Model file for the job. Use its own axes, mm. A direction names the side the tool comes from. Give positions to 0.01 mm unless a question says otherwise; leave off trailing zeros. Loops run counter-clockwise (first coordinate to the right, second up) from the corner with the lowest first, then second, coordinate; pieces in that order, holes last. Notation, with made-up numbers: M 27.25,22 L 59.25,22 A17 ccw 59.25,34 Z; hole C 5,59.25 d2. An arc over 180 degrees is marked long. Use CSV: the item, a comma, the result in double quotes. Start each with the question number.
(1) Slice it at A-A on x = -44.5. List the corners of the cut face in (y, z).
(2) Tool access for faces 1 (the face through (-17, 8, 38.069)), 2 (the face through (0, 10, -17)), 3 (the face through (-17, 11, -9.431)): list every direction of +Z, -Z, +X, -X, +Y, -Y with a clear straight run to the whole face (end or side of a thin tool).
(3) Slice it at B-B on y = 3. List the corners of the cut face in (x, z).
(4) Slice it at C-C on z = 2. List the corners of the cut face in (x, y), and give its area (3 significant figures).
(5) Flat gauge pins, fed straight in: P1, Ø6, axis at x = -45, y = 6, coming from the -Z side; P2, Ø1.2, axis at x = -16.5, z = -10.5, coming from the +Y side; P3, Ø8, axis at x = -31.5, z = -4, coming from the -Y side. Where does each tip first touch, or does it go through?
(6) Wall check: line 1 along X through (y, z) = (6.75, 35.5); line 2 along Z through (x, y) = (-50, 10.5); line 3 along Y through (x, z) = (1, 20). Give the ranges that are in metal, low to high. Write a range as from..to.
(7) Two-plate mould, pull along Z, no slides. Class faces 4 (the face through (-17, 0, 8)), 5 (the face through (-17, 8, -21.931)), 6 (the face through (-17, 11, 13.069)): pulls with the +Z half, pulls with the -Z half, needs draft (parallel to the pull), parting line crosses it, or undercut.
(8) Slice it at D-D on x = -16. List the corners of the cut face in (y, z), and give its area (3 significant figures).
```python
from build123d import *

# Parameters (mm, degrees)
CROQUIS1_W                = 10
CROQUIS1_H                = 60
SALIENTE_EXTRUIR1_DEPTH   = 10
SALIENTE_EXTRUIR1_2_DEPTH = 10
SALIENTE_EXTRUIR1_3_DEPTH = 10
CROQUIS2_W                = 80
CROQUIS2_H                = 10
SALIENTE_EXTRUIR2_DEPTH   = 2.5


with BuildPart() as part:
    # Croquis1 → Saliente-Extruir1 (new body)
    with BuildSketch(Plane(origin=(0, 0, 0), x_dir=(1, 0, 0), z_dir=(0, 1, 0))):
        with Locations((-51.849391859, -8.068789191)):
            Rectangle(CROQUIS1_W, CROQUIS1_H)
    extrude(amount=SALIENTE_EXTRUIR1_DEPTH)



with BuildPart() as body_2:
    # Croquis1 → Saliente-Extruir1 2 (new body)
    with BuildSketch(Plane(origin=(0, 0, 0), x_dir=(1, 0, 0), z_dir=(0, 1, 0))):
        with Locations((-16.849391859, -8.068789191)):
            Rectangle(CROQUIS1_W, CROQUIS1_H)
    extrude(amount=SALIENTE_EXTRUIR1_2_DEPTH)


with BuildPart() as body_3:
    # Croquis1 → Saliente-Extruir1 3 (new body)
    with BuildSketch(Plane(origin=(0, 0, 0), x_dir=(1, 0, 0), z_dir=(0, 1, 0))):
        with Locations((18.150608141, -8.068789191)):
            Rectangle(CROQUIS1_W, CROQUIS1_H)
    extrude(amount=SALIENTE_EXTRUIR1_3_DEPTH)


with BuildPart() as part_1:
    add(part.part)

    add(body_2.part)  # Saliente-Extruir2 merges body 2

    add(body_3.part)  # Saliente-Extruir2 merges body 3
    # Croquis2 → Saliente-Extruir2 (add)
    with BuildSketch(Plane(origin=(0, 10, 0), x_dir=(1, 0, 0), z_dir=(0, 1, 0))):
        with Locations((-16.849391859, -33.068789191)):
            Rectangle(CROQUIS2_W, CROQUIS2_H)
        with Locations((-16.849391859, 16.931210809)):
            Rectangle(CROQUIS2_W, CROQUIS2_H)
        with Locations((-16.849391859, 4.431210809)):
            Rectangle(CROQUIS2_W, CROQUIS2_H)
        with Locations((-16.849391859, -20.568789191)):
            Rectangle(CROQUIS2_W, CROQUIS2_H)
        with Locations((-16.849391859, -8.068789191)):
            Rectangle(CROQUIS2_W, CROQUIS2_H)
    extrude(amount=SALIENTE_EXTRUIR2_DEPTH)


solid = part_1.part
```
Reply:
1,outline,"M 10,-21.93 L 12.5,-21.93 L 12.5,-11.93 L 10,-11.93 Z; M 10,-9.43 L 12.5,-9.43 L 12.5,0.57 L 10,0.57 Z; M 10,3.07 L 12.5,3.07 L 12.5,13.07 L 10,13.07 Z; M 10,15.57 L 12.5,15.57 L 12.5,25.57 L 10,25.57 Z; M 10,28.07 L 12.5,28.07 L 12.5,38.07 L 10,38.07 Z"
2,face 1,"+Z, +X, -X, +Y, -Y"
2,face 2,"+Z, -Z, -Y"
2,face 3,"+X, -X, +Y"
3,outline,"M -56.85,-21.93 L -46.85,-21.93 L -46.85,38.07 L -56.85,38.07 Z; M -21.85,-21.93 L -11.85,-21.93 L -11.85,38.07 L -21.85,38.07 Z; M 13.15,-21.93 L 23.15,-21.93 L 23.15,38.07 L 13.15,38.07 Z"
4,outline,"M -56.85,0 L -46.85,0 L -46.85,10 L -56.85,10 Z; M -21.85,0 L -11.85,0 L -11.85,10 L -21.85,10 Z; M 13.15,0 L 23.15,0 L 23.15,10 L 13.15,10 Z"
4,area,"300 mm^2"
5,P1,"stops at z = -21.93"
5,P2,"stops at y = 10"
5,P3,"stops at y = 10"
6,line 1,"x = -56.85..-46.85, -21.85..-11.85, 13.15..23.15"
6,line 2,"z = -21.93..-11.93, -9.43..0.57, 3.07..13.07, 15.57..25.57, 28.07..38.07"
6,line 3,"y = 10..12.5"
7,face 4,"needs draft"
7,face 5,"pulls with the -Z half"
7,face 6,"undercut"
8,outline,"M 0,-21.93 L 12.5,-21.93 L 12.5,-11.93 L 10,-11.93 L 10,-9.43 L 12.5,-9.43 L 12.5,0.57 L 10,0.57 L 10,3.07 L 12.5,3.07 L 12.5,13.07 L 10,13.07 L 10,15.57 L 12.5,15.57 L 12.5,25.57 L 10,25.57 L 10,28.07 L 12.5,28.07 L 12.5,38.07 L 0,38.07 Z"
8,area,"725 mm^2"
